The listing builds one solid part. Answer for the finished solid, in the listing's coordinates (mm). A direction names the side the tool comes from. Give positions to 0.01 mm unless a question says otherwise; leave off trailing zeros. Loops run counter-clockwise (first coordinate to the right, second up) from the corner with the lowest first, then second, coordinate; pieces in that order, holes last. Notation, with made-up numbers: (41, 44.5) - (89, 44.5) arc R15 cw to (89, 65.5) - close; hole circle Ø4 at (-38, -29.5). An arc over 180 degrees is marked (long way). Write item = value, one per line. Start each with the question number.
1) Which of the six approach directions +Z, -Z, +X, -X, +Y, -Y give full straight-line access (tool end or side, diameter ignored) to faces 5 (the flat face through (12, 78.45, 12)), 6 (the flat face through (12, -78.45, 12)), 7 (the flat face through (8, 97.5, -26))?
2) Flat-ended cylindrical pins translate along their axes: P1, Ø1, axis at x = -28, y = 63, coming from the +Z side; P2, Ø1, axis at x = -0.5, y = 30, coming from the -Z side; P3, Ø3, axis at x = -6, y = 42, coming from the +Z side. Find the tip coordinate at first contact, or state that the pin passes through.
3) The part is cut by section C-C on y = 62.5. Write down the section's boundary in (x, z) (3 decimals).
4) The part is cut by section D-D on z = -24. Write down the section's boundary in (x, y), plus the area to 3 significant figures.
5) The mould has two halves that part along Z. Classify faces 1 (the cylindrical face through (-30.235, 1.365, 23.183)), 2 (the cylindrical face through (-19.89, 88.11, -18.24)), 3 (the cylindrical face through (-19.89, -88.11, -18.24)), 4 (the flat face through (8, -97.5, -26)): +Z half, -Z half, draft (parallel to the pull), parting line (faces both ways), or undercut.
6) Consider probe 1 along X at (y, z) = (27, 0) (3 decimals); probe 2 along Z at (x, y) = (0, -91.75). Determine where each line is inside the solid, lowest interval first.
7) The part is cut by section B-B on z = -12. Write down the section's boundary in (x, y).
from build123d import *

# Parameters (mm, degrees)
SKETCH1_R                = 38.1
BOSS_EXTRUDE1_DEPTH      = 97.5
BOSS_EXTRUDE1_DEPTH_BACK = 97.5
SKETCH2_R                = 26.9875
CUT_EXTRUDE1_DEPTH       = 19.05
SKETCH3_R                = 15.875
CUT_EXTRUDE2_DEPTH       = 176.95


with BuildPart() as part:
    # Sketch1 → Boss-Extrude1 (new body, two sides)
    with BuildSketch(Plane(origin=(0, 0, 0), x_dir=(1, 0, 0), z_dir=(0, 1, 0))) as boss_extrude1_sk:
        Circle(SKETCH1_R)
    extrude(amount=BOSS_EXTRUDE1_DEPTH)
    extrude(boss_extrude1_sk.sketch, amount=-BOSS_EXTRUDE1_DEPTH_BACK)

    # Sketch2 → Cut-Extrude1 (cut)
    with BuildSketch(Plane(origin=(0, 97.5, 0), x_dir=(1, 0, 0), z_dir=(0, 1, 0))):
        Circle(SKETCH2_R)
    cut_extrude1 = extrude(amount=-CUT_EXTRUDE1_DEPTH, mode=Mode.SUBTRACT)

    # Mirror1: Cut-Extrude1 across plane
    add(cut_extrude1.mirror(Plane.ZX), mode=Mode.SUBTRACT)

    # Sketch3 → Cut-Extrude2 (cut, through all)
    with BuildSketch(Plane(origin=(0, 78.45, 0), x_dir=(1, 0, 0), z_dir=(0, 1, 0))):
        Circle(SKETCH3_R)
    extrude(amount=-CUT_EXTRUDE2_DEPTH, mode=Mode.SUBTRACT)


solid = part.part
Answer below:
q1.face_5 = +Y
q1.face_6 = -Y
q1.face_7 = +Z, -Z, +X, -X, +Y
q2.P1 = 26.37
q2.P2 = -38.1
q2.P3 = 37.83
q3.outline = circle Ø76.2 at (0, 0); hole circle Ø31.75 at (0, 0)
q4.outline = (-29.59, -97.5) - (-12.34, -97.5) - (-12.34, -78.45) - (12.34, -78.45) - (12.34, -97.5) - (29.59, -97.5) - (29.59, 97.5) - (12.34, 97.5) - (12.34, 78.45) - (-12.34, 78.45) - (-12.34, 97.5) - (-29.59, 97.5) - close
q4.area = 10,600 mm2
q5.face_1 = parting line
q5.face_2 = undercut
q5.face_3 = undercut
q5.face_4 = draft
q6.probe_1 = -38.1 to -15.875, 15.875 to 38.1
q6.probe_2 = -38.1 to -26.99, 26.99 to 38.1
q7.outline = (-36.16, -97.5) - (-24.17, -97.5) - (-24.17, -78.45) - (-10.39, -78.45) - (-10.39, 78.45) - (-24.17, 78.45) - (-24.17, 97.5) - (-36.16, 97.5) - close; (10.39, -78.45) - (24.17, -78.45) - (24.17, -97.5) - (36.16, -97.5) - (36.16, 97.5) - (24.17, 97.5) - (24.17, 78.45) - (10.39, 78.45) - close
